```python
from build123d import *

# Parameters (mm, degrees)
SKETCH1_R           = 165
SKETCH1_R_2         = 100
BOSS_EXTRUDE1_DEPTH = 3.175
CUT_EXTRUDE1_DEPTH  = 3.175
CIRPATTERN1_COUNT   = 12


with BuildPart() as part:
    # Sketch1 → Boss-Extrude1 (new body)
    with BuildSketch(Plane.XY):
        Circle(SKETCH1_R)
        Circle(SKETCH1_R_2, mode=Mode.SUBTRACT)
    extrude(amount=BOSS_EXTRUDE1_DEPTH)

    # Sketch2 → Cut-Extrude1 (cut)
    with BuildSketch(Plane.XY.offset(3.175)):
        with BuildLine():
            Line((-113, 104.761860629), (7, 104.761860629))
            ThreePointArc((7, 104.761860629), (9, 102.761860629), (7, 100.761860629))
            Line((7, 100.761860629), (-113, 100.761860629))
            ThreePointArc((-113, 100.761860629), (-115, 102.761860629), (-113, 104.761860629))
        make_face()
    cut_extrude1 = extrude(amount=-CUT_EXTRUDE1_DEPTH, mode=Mode.SUBTRACT)

    # CirPattern1: Cut-Extrude1 ×12 about axis
    cirpattern1_axis = Axis((0, 0, 0), (0, 0, 1))
    for i in range(1, CIRPATTERN1_COUNT):
        add(cut_extrude1.rotate(cirpattern1_axis, i * 360 / CIRPATTERN1_COUNT), mode=Mode.SUBTRACT)


solid = part.part
```
CAD build for the part. Positions are in the model's coordinates, mm. A direction names the side the tool comes from. Round coordinates to 2 decimals unless told otherwise and drop trailing zeros. Order: outer loops, then holes, each group sorted by start corner. A loop starts at its lowest first (then second) coordinate and runs counter-clockwise, first axis right, second up.
Q1. Two-plate mould, pull along X, no slides. Class faces 1 (the flat face through (95.553, -61.182, 1.61)), 2 (the flat face through (71, -71, 0)), 3 (the cylindrical face through (-35.769, -161.076, 1.565)): pulls with the +X half, pulls with the -X half, needs draft (parallel to the pull), parting line crosses it, or undercut.
Q2. Slice it at D-D (x = -64). Write the cut outline in (y, z) (1 decimal), and give its area (3 significant figures).
Q3. Slice it at A-A (y = 138). Write the cut outline in (x, z) (3 decimals), and give its area (3 significant figures).
Q4. Which spindle directions (+Z, -Z, +X, -X, +Y, -Y) get a long thin tool onto all of the face, cutting with end or side? Do faces 4 (the flat face through (71, -71, 3.175)), 5 (the flat face through (-113.34, 5.21, 1.61)). Say none if no direction does.
Q5. Slice it at B-B (x = 0). Write the cut outline in (y, z) (3 decimals).
Q6. Drop flat-ended pins along their axis: pin 1 (1.6 mm diameter, centred on x = 58, z = 2, fed in from -Y); pin 2 (1.5 mm diameter, centred on x = 41, z = 1, fed in from -Y); pin 3 (1.6 mm diameter, centred on y = -71.5, z = 1, fed in from -X); pin 4 (1 mm diameter, centred on x = 101.5, y = 28.5, fed in from -Z). Give the stop position or say it passes through.
Q7. Wall check: L1, parallel to Y at x = 89.5, z = 2.4; L2, parallel to Y at x = 59.5, z = 1.4; L3, parallel to Y at x = 0, z = 1.3. Give the ranges that are in metal, low to high.
Q8. Slice it at C-C (y = -69). Write the cut outline in (x, z) (3 decimals), and give its area (3 significant figures).
Results below:
1. face 1: undercut
1. face 2: needs draft
1. face 3: parting line crosses it
2. outline: (-152.1, 0) - (-98.7, 0) - (-98.7, 3.2) - (-152.1, 3.2) - close; (-90.7, 0) - (-76.8, 0) - (-76.8, 3.2) - (-90.7, 3.2) - close; (76.8, 0) - (79.4, 0) - (79.4, 3.2) - (76.8, 3.2) - close; (84, 0) - (100.8, 0) - (100.8, 3.2) - (84, 3.2) - close; (104.8, 0) - (152.1, 0) - (152.1, 3.2) - (104.8, 3.2) - close
2. area: 425 mm2
3. outline: (-90.449, 0) - (-37.499, 0) - (-37.499, 3.175) - (-90.449, 3.175) - close; (-29.499, 0) - (36.675, 0) - (36.675, 3.175) - (-29.499, 3.175) - close; (41.294, 0) - (90.449, 0) - (90.449, 3.175) - (41.294, 3.175) - close
3. area: 534 mm2
4. face 4: +Z, +X, -X, +Y, -Y
4. face 5: +Z, -Z
5. outline: (-165, 0) - (-120.969, 0) - (-120.969, 3.175) - (-165, 3.175) - close; (-116.35, 0) - (-104.762, 0) - (-104.762, 3.175) - (-116.35, 3.175) - close; (-100.762, 0) - (-100, 0) - (-100, 3.175) - (-100.762, 3.175) - close; (100, 0) - (100.762, 0) - (100.762, 3.175) - (100, 3.175) - close; (104.762, 0) - (116.35, 0) - (116.35, 3.175) - (104.762, 3.175) - close; (120.969, 0) - (165, 0) - (165, 3.175) - (120.969, 3.175) - close
6. pin 1: stops at y = -154.77
6. pin 2: stops at y = -160.02
6. pin 3: stops at x = -149.09
6. pin 4: passes through
7. L1: y = -138.62 to -104.76, -100.76 to -69.3, -64.68 to -54.51, -46.51 to -44.61, 44.61 to 46.51, 54.51 to 138.62
7. L2: y = -153.9 to -104.76, -100.76 to -86.62, -82 to -80.37, 80.37 to 98.47, 106.47 to 153.9
7. L3: y = -165 to -120.97, -116.35 to -104.76, -100.76 to -100, 100 to 100.76, 104.76 to 116.35, 120.97 to 165
8. outline: (-149.88, 0) - (-104.762, 0) - (-104.762, 3.175) - (-149.88, 3.175) - close; (-100.762, 0) - (-81.131, 0) - (-81.131, 3.175) - (-100.762, 3.175) - close; (-76.513, 0) - (-72.381, 0) - (-72.381, 3.175) - (-76.513, 3.175) - close; (72.381, 0) - (82.012, 0) - (82.012, 3.175) - (72.381, 3.175) - close; (90.012, 0) - (149.88, 0) - (149.88, 3.175) - (90.012, 3.175) - close
8. area: 439 mm2
